from build123d import *

# Parameters (mm, degrees)
F0_W     = 305
F0_H     = 305
F1_DEPTH = 21
F2_R     = 20
F3_DEPTH = 130


with BuildPart() as f1:
    # F0 (on Front) → F1 (new body, symmetric)
    with BuildSketch(Plane.XZ):
        Rectangle(F0_W, F0_H)
    extrude(amount=F1_DEPTH, both=True)

    # F2 (on face) → F3 (join)
    with BuildSketch(Plane.XY.offset(152.5)):
        Circle(F2_R)
    extrude(amount=F3_DEPTH)


solid = f1.part
Source: CAD feature listing. Evaluate the final solid. Frame: model axes, mm. A direction names the side the tool comes from. Coordinates: 2 decimals unless noted, no trailing zeros. Order: outer loops, then holes, each group sorted by start corner. A loop starts at its lowest first (then second) coordinate and runs counter-clockwise, first axis right, second up. Notation, with made-up numbers: M -16,6.5 L 25,6.5 A27 cw 25,34.5 Z; hole C 82.25,-16.75 d1. An arc over 180 degrees is marked long. Write each question's results on one line, items separated by ' | '. Start each with the question number.
1. Reachability of faces 1 (the face through (152.5, 0, -2)), 2 (the face through (-4.336, -19.524, 216.59)) from +Z, -Z, +X, -X, +Y, -Y: full face, straight path, thin tool, end or side. Return the list, or none.
2. Section C-C, the plane z = 194. Return the cut outline in (x, y).
3. Material intervals for L1, parallel to Z at x = -53.5, y = -16.5; L2, parallel to X at y = 1, z = 256; L3, parallel to X at y = 5, z = 242, sorted ascending.
4. Section D-D, the plane x = 2. Return the cut outline in (y, z).
5. Section B-B, the plane x = -82. Return the cut outline in (y, z).
6. Section A-A, the plane y = 0. Return the cut outline in (x, z).
7. Pin query (flat end, axial travel): pin 1 (12 mm diameter, centred on y = 1, z = 218.5, fed in from -X); pin 2 (2 mm diameter, centred on x = 28, y = 13, fed in from +Z). Return the tip coordinate at first contact, or that it passes through.
Solution:
1) face 1: +Z, -Z, +X, +Y, -Y | face 2: +Z
2) outline: C 0,0 d40
3) L1: -152.5 to 152.5 | L2: -19.97 to 19.97 | L3: -19.36 to 19.36
4) outline: M -21,-152.5 L 21,-152.5 L 21,152.5 L 19.9,152.5 L 19.9,282.5 L -19.9,282.5 L -19.9,152.5 L -21,152.5 Z
5) outline: M -21,-152.5 L 21,-152.5 L 21,152.5 L -21,152.5 Z
6) outline: M -152.5,-152.5 L 152.5,-152.5 L 152.5,152.5 L 20,152.5 L 20,282.5 L -20,282.5 L -20,152.5 L -152.5,152.5 Z
7) pin 1: x = -20 | pin 2: z = 152.5
